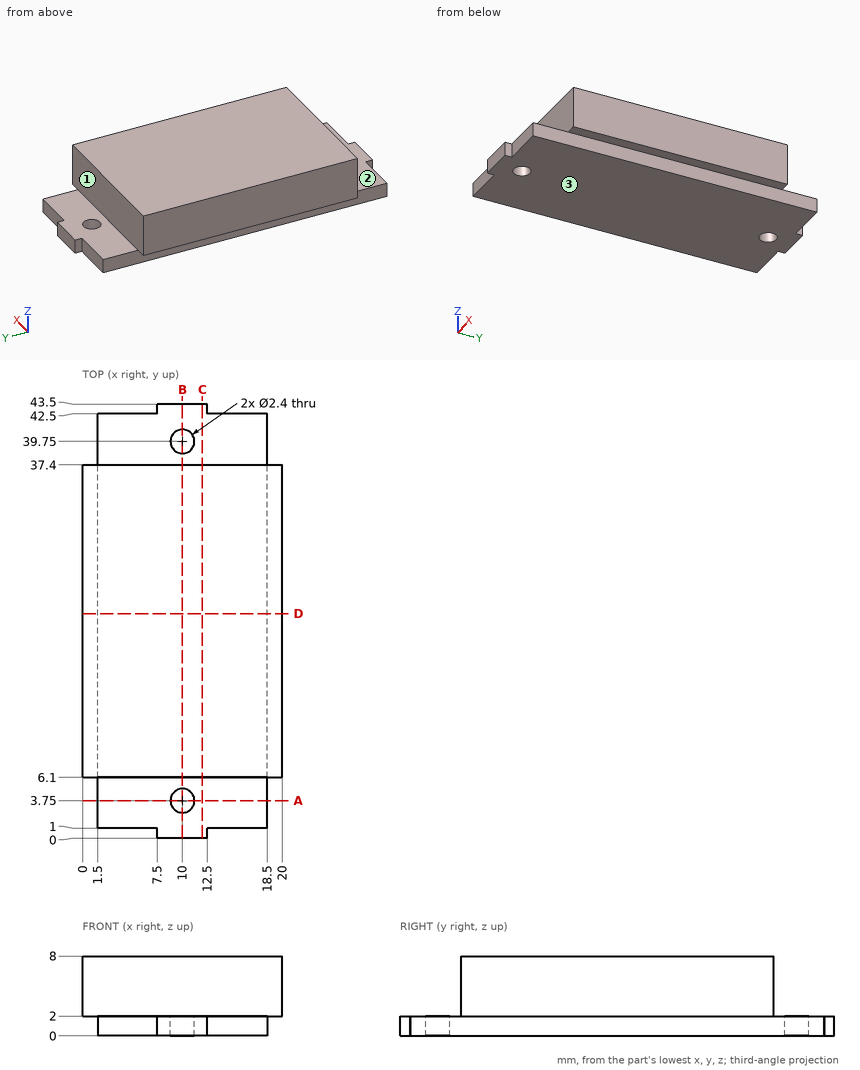
Job drawing, mm, ordinate dimensions from the low corner. One solid piece. A direction names the side the tool comes from. Round coordinates to 2 decimals unless told otherwise and drop trailing zeros. Write each loop counter-clockwise with the first axis right and the second up, starting at its lowest first coordinate (ties: lowest second). Pieces come first, ordered by that corner, then holes. Notation, with made-up numbers: (-5, -31) -> (4, -31) arc R18 ccw to (4, -5) -> close; hole circle Ø1 at (59.5, 7.5). An arc over 180 degrees is marked (long way). Answer as a JSON object with one key per item and string values.
(1) Band-saw the part on C-C, the plane x = 12. List the corners of the cut face in (y, z).
Reported:
{"outline": "(0, 0) -> (43.5, 0) -> (43.5, 2) -> (37.4, 2) -> (37.4, 8) -> (6.1, 8) -> (6.1, 2) -> (0, 2) -> close"}
(2) Probe probe 1 along Y at (x, z) = (10, 0.8); probe 2 along X at (y, z) = (39.75, 1.45); probe 3 along Y at (x, z) = (9, 0.5). List the from-to ranges inside material, lowest first. Write a range as [from, to].
Reported:
{"probe 1": "y = [0, 2.55], [4.95, 38.55], [40.95, 43.5]", "probe 2": "x = [1.5, 8.8], [11.2, 18.5]", "probe 3": "y = [0, 3.09], [4.41, 39.09], [40.41, 43.5]"}
(3) Pin check, flat tips, straight feed: P1, Ø5, axis at x = 8.5, y = 40.5, coming from the +Z side; P2, Ø4, axis at x = 10, y = 3.75, coming from the -Z side; P3, Ø0.6, axis at y = 32, z = 1, coming from the -X side; P4, Ø0.5, axis at y = 43, z = 1.5, coming from the -X side. Stop position of each tip, or through.
Reported:
{"P1": "stops at z = 2", "P2": "stops at z = 0", "P3": "stops at x = 1.5", "P4": "stops at x = 7.5"}
(4) Band-saw the part on A-A, the plane y = 3.75. List the corners of the cut face in (x, z).
Reported:
{"outline": "(1.5, 0) -> (8.8, 0) -> (8.8, 2) -> (1.5, 2) -> close; (11.2, 0) -> (18.5, 0) -> (18.5, 2) -> (11.2, 2) -> close"}
(5) Band-saw the part on D-D, the plane y = 22.5. List the corners of the cut face in (x, z).
Reported:
{"outline": "(0, 2) -> (1.5, 2) -> (1.5, 0) -> (18.5, 0) -> (18.5, 2) -> (20, 2) -> (20, 8) -> (0, 8) -> close"}
(6) Band-saw the part on B-B, the plane x = 10. List the corners of the cut face in (y, z).
Reported:
{"outline": "(0, 0) -> (2.55, 0) -> (2.55, 2) -> (0, 2) -> close; (4.95, 0) -> (38.55, 0) -> (38.55, 2) -> (37.4, 2) -> (37.4, 8) -> (6.1, 8) -> (6.1, 2) -> (4.95, 2) -> close; (40.95, 0) -> (43.5, 0) -> (43.5, 2) -> (40.95, 2) -> close"}
(7) Which spindle directions (+Z, -Z, +X, -X, +Y, -Y) get a long thin tool onto all of the face, cutting with end or side? Do the marked faces 1, 2 and 3. Say none if no direction does.
Reported:
{"face 1": "+Z, +X, -X, +Y", "face 2": "+Z, +X, -X, -Y", "face 3": "-Z, +X, -X, +Y, -Y"}
